```python
from build123d import *

# Parameters (mm, degrees)
SKETCH1_W           = 37
SKETCH1_H           = 13.5
BOSS_EXTRUDE1_DEPTH = 15.5
SKETCH2_W           = 24
SKETCH2_H           = 21
CUT_EXTRUDE1_DEPTH  = 31
SKETCH3_W           = 24
SKETCH3_H           = 27
BOSS_EXTRUDE2_DEPTH = 1.25
SKETCH4_W           = 24
SKETCH4_H           = 27
BOSS_EXTRUDE3_DEPTH = 1.25
SKETCH5_W           = 24
SKETCH5_H           = 27
BOSS_EXTRUDE4_DEPTH = 0.625
CUT_EXTRUDE2_DEPTH  = 30
CUT_EXTRUDE3_DEPTH  = 30
BOSS_EXTRUDE5_DEPTH = 10
SKETCH9_W           = 13.5
SKETCH9_H           = 12
BOSS_EXTRUDE6_DEPTH = 0.75
CUT_EXTRUDE6_START  = -0.75
CUT_EXTRUDE6_DEPTH  = 0.75
CUT_EXTRUDE7_DEPTH  = 0.75
SKETCH15_W          = 13.5
SKETCH15_H          = 12
BOSS_EXTRUDE7_DEPTH = 0.75
CUT_EXTRUDE8_START  = -0.75
CUT_EXTRUDE8_DEPTH  = 0.75
CUT_EXTRUDE9_DEPTH  = 0.75


# Read off the part's stored shape, not the designer's step: Cut-Extrude6, Cut-Extrude8
with BuildPart() as part:
    # Sketch1 → Boss-Extrude1 (new, symmetric)
    with BuildSketch(Plane.XY):
        Rectangle(SKETCH1_W, SKETCH1_H)
    extrude(amount=BOSS_EXTRUDE1_DEPTH, both=True)

    # Sketch2 → Cut-Extrude1 (cut)
    with BuildSketch(Plane(origin=(0, 6.75, 0), x_dir=(1, 0, 0), z_dir=(0, 1, 0))):
        Rectangle(SKETCH2_W, SKETCH2_H)
    extrude(amount=-CUT_EXTRUDE1_DEPTH, mode=Mode.SUBTRACT)

    # Sketch3 → Boss-Extrude2 (add)
    with BuildSketch(Plane.XY.offset(-10.5)):
        Rectangle(SKETCH3_W, SKETCH3_H)
    extrude(amount=BOSS_EXTRUDE2_DEPTH)

    # Sketch4 → Boss-Extrude3 (add)
    with BuildSketch(Plane(origin=(0, 0, 10.5), x_dir=(-1, 0, 0), z_dir=(0, 0, -1))):
        Rectangle(SKETCH4_W, SKETCH4_H)
    extrude(amount=BOSS_EXTRUDE3_DEPTH)

    # Sketch5 → Boss-Extrude4 (add, symmetric)
    with BuildSketch(Plane.XY):
        Rectangle(SKETCH5_W, SKETCH5_H)
    extrude(amount=BOSS_EXTRUDE4_DEPTH, both=True)

    # Sketch6 → Cut-Extrude2 (cut)
    with BuildSketch(Plane(origin=(0, 0, -10.5), x_dir=(-1, 0, 0), z_dir=(0, 0, -1))):
        with BuildLine():
            Line((-12, -13.5), (-12, -11))
            ThreePointArc((-12, -11), (-11.267766953, -12.767766953), (-9.5, -13.5))
            Line((-9.5, -13.5), (-12, -13.5))
        make_face()
        with BuildLine():
            Line((12, -13.5), (12, -11))
            ThreePointArc((12, -11), (11.267766953, -12.767766953), (9.5, -13.5))
            Line((9.5, -13.5), (12, -13.5))
        make_face()
    extrude(amount=-CUT_EXTRUDE2_DEPTH, mode=Mode.SUBTRACT)

    # Sketch7 → Cut-Extrude3 (cut)
    with BuildSketch(Plane(origin=(0, 0, -10.5), x_dir=(-1, 0, 0), z_dir=(0, 0, -1))):
        with BuildLine():
            Line((12, 13.5), (9.5, 13.5))
            ThreePointArc((9.5, 13.5), (11.267766953, 12.767766953), (12, 11))
            Line((12, 11), (12, 13.5))
        make_face()
        with BuildLine():
            Line((-12, 13.5), (-12, 11))
            ThreePointArc((-12, 11), (-11.267766953, 12.767766953), (-9.5, 13.5))
            Line((-9.5, 13.5), (-12, 13.5))
        make_face()
    extrude(amount=-CUT_EXTRUDE3_DEPTH, mode=Mode.SUBTRACT)

    # Sketch8 → Boss-Extrude5 (add, symmetric)
    with BuildSketch(Plane.XY):
        with BuildLine():
            Line((-5.5, 12), (5.5, 12))
            ThreePointArc((5.5, 12), (9.035533906, 10.535533906), (10.5, 7))
            Line((10.5, 7), (10.5, -7))
            ThreePointArc((10.5, -7), (9.035533906, -10.535533906), (5.5, -12))
            Line((5.5, -12), (-5.5, -12))
            ThreePointArc((-5.5, -12), (-9.035533906, -10.535533906), (-10.5, -7))
            Line((-10.5, -7), (-10.5, 7))
            ThreePointArc((-10.5, 7), (-9.035533906, 10.535533906), (-5.5, 12))
        make_face()
    extrude(amount=BOSS_EXTRUDE5_DEPTH, both=True)

    # Sketch9 → Boss-Extrude6 (add)
    with BuildSketch(Plane(origin=(0, 0, -15.5), x_dir=(0, -1, 0), z_dir=(0, 0, -1))):
        with Locations((0, 24.5)):
            Rectangle(SKETCH9_W, SKETCH9_H)
    extrude(amount=-BOSS_EXTRUDE6_DEPTH)

    # Cut-Extrude6 outline → Cut-Extrude6 (cut)
    with BuildSketch(Plane.XY.offset(-14.75).offset(CUT_EXTRUDE6_START)):
        with BuildLine():
            Line((-30.5, 6.75), (-30.5, 1.75))
            ThreePointArc((-30.5, 1.75), (-29.035533906, 5.285533906), (-25.5, 6.75))
            Line((-25.5, 6.75), (-30.5, 6.75))
        make_face()
        with BuildLine():
            ThreePointArc((-25.5, -6.75), (-29.035533906, -5.285533906), (-30.5, -1.75))
            Line((-30.5, -1.75), (-30.5, -6.75))
            Line((-30.5, -6.75), (-25.5, -6.75))
        make_face()
    extrude(amount=CUT_EXTRUDE6_DEPTH, mode=Mode.SUBTRACT)

    # Sketch14 → Cut-Extrude7 (cut)
    with BuildSketch(Plane.XY.offset(-14.75)):
        with BuildLine():
            Line((-25.95, 1.725), (-23.05, 1.725))
            ThreePointArc((-23.05, 1.725), (-21.847918472, 1.227081528), (-21.35, 0.025))
            Line((-21.35, 0.025), (-21.35, -0.025))
            ThreePointArc((-21.35, -0.025), (-21.847918472, -1.227081528), (-23.05, -1.725))
            Line((-23.05, -1.725), (-25.95, -1.725))
            ThreePointArc((-25.95, -1.725), (-27.152081528, -1.227081528), (-27.65, -0.025))
            Line((-27.65, -0.025), (-27.65, 0.025))
            ThreePointArc((-27.65, 0.025), (-27.152081528, 1.227081528), (-25.95, 1.725))
        make_face()
    extrude(amount=-CUT_EXTRUDE7_DEPTH, mode=Mode.SUBTRACT)

    # Sketch15 → Boss-Extrude7 (add)
    with BuildSketch(Plane.YX.offset(15.5)):
        with Locations((0, 24.5)):
            Rectangle(SKETCH15_W, SKETCH15_H)
    extrude(amount=-BOSS_EXTRUDE7_DEPTH)

    # Cut-Extrude8 outline → Cut-Extrude8 (cut)
    with BuildSketch(Plane.XY.offset(-14.75).offset(CUT_EXTRUDE8_START)):
        with BuildLine():
            Line((30.5, -6.75), (30.5, -1.75))
            ThreePointArc((30.5, -1.75), (29.035533906, -5.285533906), (25.5, -6.75))
            Line((25.5, -6.75), (30.5, -6.75))
        make_face()
        with BuildLine():
            ThreePointArc((25.5, 6.75), (29.035533906, 5.285533906), (30.5, 1.75))
            Line((30.5, 1.75), (30.5, 6.75))
            Line((30.5, 6.75), (25.5, 6.75))
        make_face()
    extrude(amount=CUT_EXTRUDE8_DEPTH, mode=Mode.SUBTRACT)

    # Sketch18 → Cut-Extrude9 (cut)
    with BuildSketch(Plane.XY.offset(-14.75)):
        with BuildLine():
            Line((23.05, 1.725), (25.95, 1.725))
            ThreePointArc((25.95, 1.725), (27.152081528, 1.227081528), (27.65, 0.025))
            Line((27.65, 0.025), (27.65, -0.025))
            ThreePointArc((27.65, -0.025), (27.152081528, -1.227081528), (25.95, -1.725))
            Line((25.95, -1.725), (23.05, -1.725))
            ThreePointArc((23.05, -1.725), (21.847918472, -1.227081528), (21.35, -0.025))
            Line((21.35, -0.025), (21.35, 0.025))
            ThreePointArc((21.35, 0.025), (21.847918472, 1.227081528), (23.05, 1.725))
        make_face()
    extrude(amount=-CUT_EXTRUDE9_DEPTH, mode=Mode.SUBTRACT)


solid = part.part
```
CAD build for the part. Positions are in the model's coordinates, mm. A direction names the side the tool comes from. Round coordinates to 2 decimals unless told otherwise and drop trailing zeros. Write each loop counter-clockwise with the first axis right and the second up, starting at its lowest first coordinate (ties: lowest second). Pieces come first, ordered by that corner, then holes. Notation, with made-up numbers: (-19, 38) -> (35, 38) arc R17 ccw to (35, 52) -> close; hole circle Ø11 at (36, 48). An arc over 180 degrees is marked (long way). Answer in a Markdown table with one row per item. Add a question column.
Item 1: Which spindle directions (+Z, -Z, +X, -X, +Y, -Y) get a long thin tool onto all of the face, cutting with end or side? Do faces 4 (the face through (-9, -10.57, -4.88)), 5 (the face through (-12, -9, 10)), 6 (the face through (12, -9, -10)), 7 (the face through (-11, 0, 0.625)), 8 (the face through (0, -12, 5)). Say none if no direction does.
Item 2: Drill centre lines: line 1 (Z direction, x = -6.5, y = -12.5) (3 decimals); line 2 (X direction, y = 3, z = 2); line 3 (X direction, y = -3.25, z = -11.5). Where is each one in solid material? Low to high. Write a range as from..to.
Item 3: Saw through at D-D, the plane y = -3. Write the cut outline in (x, z) (3 decimals).
Item 4: Drop flat-ended pins along their axis: pin 1 Ø2.5 at (y, z) = (1.5, -4.5) entering from +X; pin 2 Ø3.5 at (x, y) = (3, -11) entering from -Z; pin 3 Ø0.6 at (y, z) = (-9.5, 10) entering from -X; pin 4 Ø4 at (x, y) = (20.5, 10) entering from -Z. Give the stop position or say it passes through.
Item 5: Mould opens along Z. For faces 1 (the face through (-11, -13, 10)), 2 (the face through (0, 12, -5)), 3 (the face through (0, 0, -15.5)) say: pulls with the +Z half, pulls with the -Z half, needs draft (parallel to the pull), parting line crosses it, or undercut.
Item 6: Saw through at C-C, the plane y = 5.5. Write the cut outline in (x, z) (3 decimals), then the cut area to 3 significant figures.
Item 7: Saw through at B-B, the plane x = 4.5. Write the cut outline in (y, z) (3 decimals), then the cut area to 3 significant figures.
Item 8: Saw through at A-A, the plane z = 3. Write the cut outline in (x, y), then the cut area to 3 significant figures.
Findings below:
| question | item | result |
|---|---|---|
| 1 | face 4 | -X, -Y |
| 1 | face 5 | +Z, -Z, -X, -Y |
| 1 | face 6 | +Z, -Z, +X, -Y |
| 1 | face 7 | none |
| 1 | face 8 | +X, -X, -Y |
| 2 | line 1 | z = -10.5..-9.25, -0.625..0.625, 9.25..10.5 |
| 2 | line 2 | x = -18.5..-12, -10.5..10.5, 12..18.5 |
| 2 | line 3 | x = -18.5..18.5 |
| 3 | outline | (-30.341, -15.5) -> (30.341, -15.5) -> (30.341, -14.75) -> (18.5, -14.75) -> (18.5, 15.5) -> (-18.5, 15.5) -> (-18.5, -14.75) -> (-30.341, -14.75) -> close; hole (-12, -9.25) -> (-10.5, -9.25) -> (-10.5, -0.625) -> (-12, -0.625) -> close; hole (-12, 0.625) -> (-10.5, 0.625) -> (-10.5, 9.25) -> (-12, 9.25) -> close; hole (10.5, -9.25) -> (12, -9.25) -> (12, -0.625) -> (10.5, -0.625) -> close; hole (10.5, 0.625) -> (12, 0.625) -> (12, 9.25) -> (10.5, 9.25) -> close |
| 4 | pin 1 | stops at x = 18.5 |
| 4 | pin 2 | stops at z = -10.5 |
| 4 | pin 3 | stops at x = -12 |
| 4 | pin 4 | passes through |
| 5 | face 1 | needs draft |
| 5 | face 2 | undercut |
| 5 | face 3 | pulls with the -Z half |
| 6 | outline | (-28.807, -15.5) -> (28.807, -15.5) -> (28.807, -14.75) -> (18.5, -14.75) -> (18.5, 15.5) -> (-18.5, 15.5) -> (-18.5, -14.75) -> (-28.807, -14.75) -> close; hole (-12, -9.25) -> (-10.5, -9.25) -> (-10.5, -0.625) -> (-12, -0.625) -> close; hole (-12, 0.625) -> (-10.5, 0.625) -> (-10.5, 9.25) -> (-12, 9.25) -> close; hole (10.5, -9.25) -> (12, -9.25) -> (12, -0.625) -> (10.5, -0.625) -> close; hole (10.5, 0.625) -> (12, 0.625) -> (12, 9.25) -> (10.5, 9.25) -> close |
| 6 | area | 1,110 mm^2 |
| 7 | outline | (-13.5, -10.5) -> (-6.75, -10.5) -> (-6.75, -15.5) -> (6.75, -15.5) -> (6.75, -10.5) -> (13.5, -10.5) -> (13.5, -9.25) -> (12, -9.25) -> (12, -0.625) -> (13.5, -0.625) -> (13.5, 0.625) -> (12, 0.625) -> (12, 9.25) -> (13.5, 9.25) -> (13.5, 10.5) -> (6.75, 10.5) -> (6.75, 15.5) -> (-6.75, 15.5) -> (-6.75, 10.5) -> (-13.5, 10.5) -> (-13.5, 9.25) -> (-12, 9.25) -> (-12, 0.625) -> (-13.5, 0.625) -> (-13.5, -0.625) -> (-12, -0.625) -> (-12, -9.25) -> (-13.5, -9.25) -> close |
| 7 | area | 650 mm^2 |
| 8 | outline | (-18.5, -6.75) -> (-12, -6.75) -> (-12, 6.75) -> (-18.5, 6.75) -> close; (-10.5, -7) arc R5 ccw to (-5.5, -12) -> (5.5, -12) arc R5 ccw to (10.5, -7) -> (10.5, 7) arc R5 ccw to (5.5, 12) -> (-5.5, 12) arc R5 ccw to (-10.5, 7) -> close; (12, -6.75) -> (18.5, -6.75) -> (18.5, 6.75) -> (12, 6.75) -> close |
| 8 | area | 658 mm^2 |
